```python
from build123d import *

# Parameters (mm, degrees)
SKETCH2_R           = 25.4
SKETCH2_R_2         = 20.955
BOSS_EXTRUDE1_DEPTH = 3.048
SKETCH3_W           = 6.35
SKETCH3_H           = 49.944808163
BOSS_EXTRUDE2_DEPTH = 3.048
CUT_EXTRUDE1_DEPTH  = 3.302
BOSS_EXTRUDE3_DEPTH = 3.048
CUT_EXTRUDE2_DEPTH  = 3.048
SKETCH12_W          = 13.143188689
SKETCH12_H          = 6.35
BOSS_EXTRUDE5_DEPTH = 3.048
SKETCH6_W           = 27.175313858
SKETCH6_H           = 4.151974609
CUT_EXTRUDE4_DEPTH  = 3.048
BOSS_EXTRUDE6_DEPTH = 3.048


with BuildPart() as part:
    # Sketch2 → Boss-Extrude1 (new body)
    with BuildSketch(Plane.XY):
        Circle(SKETCH2_R)
        Circle(SKETCH2_R_2, mode=Mode.SUBTRACT)
    extrude(amount=BOSS_EXTRUDE1_DEPTH)

    # Sketch3 → Boss-Extrude2 (add)
    with BuildSketch(Plane.XY):
        with Locations((8.763, 6.269595919)):
            Rectangle(SKETCH3_W, SKETCH3_H)
    extrude(amount=BOSS_EXTRUDE2_DEPTH)

    # Sketch8 → Cut-Extrude1 (cut)
    with BuildSketch(Plane.XY):
        Polygon((-11.882255203, 0.183619794), (-24.319009678, -26.162), (-14.01620416, -31.025558483), (-1.579449685, -4.679938689), align=None)
    extrude(amount=CUT_EXTRUDE1_DEPTH, mode=Mode.SUBTRACT)

    # Sketch7 → Boss-Extrude3 (add)
    with BuildSketch(Plane.XY):
        Polygon((5.588, 31.242), (-21.510222, -26.162), (-15.801284542, -28.856969943), (11.296937458, 28.547030057), align=None)
    extrude(amount=BOSS_EXTRUDE3_DEPTH)

    # Sketch9 → Cut-Extrude2 (cut)
    with BuildSketch(Plane.XY):
        Polygon((5.588, -18.702808163), (5.588, 2.236396155), (16.057602159, -8.233206004), align=None)
    extrude(amount=CUT_EXTRUDE2_DEPTH, mode=Mode.SUBTRACT)

    # Sketch12 → Boss-Extrude5 (add)
    with BuildSketch(Plane.XY):
        Polygon((5.588, -15.110705714), (5.588, -1.355706294), (12.46549971, -8.233206004), align=None)
        with Locations((-0.983594345, -8.213706294)):
            Rectangle(SKETCH12_W, SKETCH12_H)
    extrude(amount=BOSS_EXTRUDE5_DEPTH)

    # Sketch6 → Cut-Extrude4 (cut)
    with BuildSketch(Plane.XY):
        with Locations((-13.587656929, -28.237987305)):
            Rectangle(SKETCH6_W, SKETCH6_H)
    extrude(amount=CUT_EXTRUDE4_DEPTH, mode=Mode.SUBTRACT)

    # Sketch13 → Boss-Extrude6 (add)
    with BuildSketch(Plane.XY):
        with BuildLine():
            Line((5.588, 31.242), (8.128, 31.242))
            ThreePointArc((8.128, 31.242), (8.763, 36.706884628), (9.398, 31.242))
            Line((9.398, 31.242), (11.938, 31.242))
            ThreePointArc((11.938, 31.242), (8.763, 38.102476668), (5.588, 31.242))
        make_face()
    extrude(amount=BOSS_EXTRUDE6_DEPTH)


solid = part.part
```
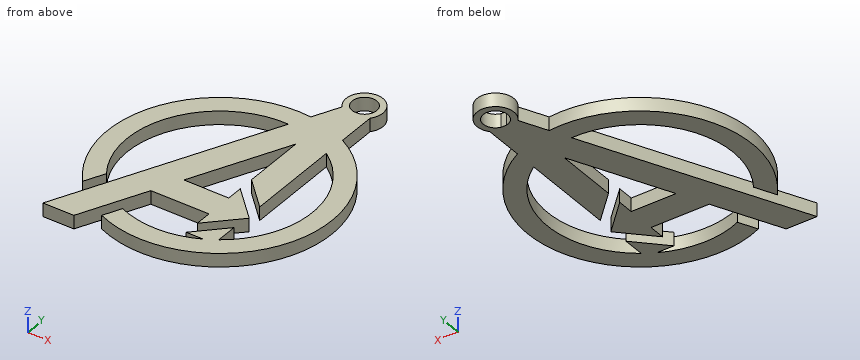
Read the model definition and answer for the solid it produces. Units are mm, in the model's axes. Give positions to 0.01 mm unless a question says otherwise; leave off trailing zeros. Order: outer loops, then holes, each group sorted by start corner. A loop starts at its lowest first (then second) coordinate and runs counter-clockwise, first axis right, second up. Notation, with made-up numbers: (33.25, 85.25) -> (50.25, 85.25) arc R14 ccw to (50.25, 90.25) -> close; hole circle Ø1 at (-17, 3.25). An arc over 180 degrees is marked (long way). One line per item, written item: value. Start each with the question number.
(1) Straight lines are drawn through the part: L1, parallel to Y at x = -7, z = 1.4; L2, parallel to Y at x = 2, z = 0.3; L3, parallel to X at y = 13, z = 1.1. For each, find the intervals that lie inside material, in ascending order.
(2) Flat-ended cylindrical pins translate along their axes: P1, Ø1.5, axis at y = -2.5, z = 1.5, coming from the -X side; P2, Ø1.5, axis at x = 0.5, z = 2, coming from the +Y side; P3, Ø0.9, axis at y = -15.5, z = 1, coming from the +X side. Find the tip coordinate at first contact, or state that the pin passes through.
(3) The part is cut by section A-A (z = 0.75). Determine the outline of the cut face in (x, y) (1 decimal).
(4) The part is cut by section C-C (y = 0). Determine the outline of the cut face in (x, z) (3 decimals), and give its area (3 significant figures).
(5) The part is cut by section D-D (x = 19). Determine the outline of the cut face in (y, z).
(6) The part is cut by section B-B (x = 1.5). Determine the outline of the cut face in (y, z), and give its area (3 significant figures).
Taken from the geometry:
1. L1: -24.42 to -19.75, -11.39 to 4.58, 19.75 to 24.42
1. L2: -25.32 to -20.86, -11.39 to -5.04, 8.85 to 25.32
1. L3: -21.82 to -16.44, -3.02 to 3.96, 5.59 to 11.94, 16.44 to 21.82
2. P1: x = -25.34
2. P2: y = 25.4
2. P3: x = 20.46
3. outline: (-21.5, -26.2) -> (-14.5, -26.2) -> (-7.6, -11.4) -> (5.6, -11.4) -> (5.6, -15.1) -> (12.5, -8.2) -> (5.6, -1.4) -> (5.6, -5) -> (-4.6, -5) -> (5.6, 16.5) -> (5.6, 2.2) -> (11.9, -4.1) -> (11.9, 17.2) arc R21 cw to (11.9, -17.2) -> (11.9, -12.4) -> (5.6, -18.7) -> (9.5, -18.7) arc R21 cw to (-8.4, -19.2) -> (-10.3, -23.2) arc R25.4 ccw to (11.9, 22.4) -> (11.9, 31.2) arc R4.2 ccw (long way) to (5.6, 31.2) -> (2.8, 25.2) arc R25.4 ccw to (-19.6, -16.2) -> (-17.4, -11.6) arc R21 cw to (0.7, 20.9) -> close; hole (8.1, 31.2) -> (9.4, 31.2) arc R2.8 ccw (long way) to start
4. outline: (-25.4, 0) -> (-20.955, 0) -> (-20.955, 3.048) -> (-25.4, 3.048) -> close; (-9.16, 0) -> (-2.179, 0) -> (-2.179, 3.048) -> (-9.16, 3.048) -> close; (7.824, 0) -> (11.938, 0) -> (11.938, 3.048) -> (7.824, 3.048) -> close; (20.955, 0) -> (25.4, 0) -> (25.4, 3.048) -> (20.955, 3.048) -> close
4. area: 60.9 mm^2
5. outline: (-16.86, 0) -> (-8.84, 0) -> (-8.84, 3.05) -> (-16.86, 3.05) -> close; (8.84, 0) -> (16.86, 0) -> (16.86, 3.05) -> (8.84, 3.05) -> close
6. outline: (-25.36, 0) -> (-20.9, 0) -> (-20.9, 3.05) -> (-25.36, 3.05) -> close; (-11.39, 0) -> (-5.04, 0) -> (-5.04, 3.05) -> (-11.39, 3.05) -> close; (7.79, 0) -> (25.36, 0) -> (25.36, 3.05) -> (7.79, 3.05) -> close
6. area: 86.5 mm^2
